Autodesk Fusion 360 part; units mm, degrees
sketch "Skizze1" plane through (0, 0, 0) normal (0, 0, 1) x (1, 0, 0)
  line L0 (-48.5045, 60.0252) -> (-48.5045, -50)
  line L1 (21.4307, 60.0126) -> (21.4307, -50)
  line L2 (-41.5077, 135.8568) -> (-13.5563, 144.0233)
  line L3 (-13.5563, 144.0233) -> (14.4793, 135.8568)
  line L4 (-41.4821, -125.8001) -> (-13.5254, -133.9377)
  line L5 (-13.5254, -133.9377) -> (14.4312, -125.8001)
  line L6 (14.4312, -125.8001) -> (14.4312, -57)
  line L7 (-41.4821, -125.8001) -> (-41.4821, -57)
  line L8 (-41.5077, 135.8568) -> (-41.5077, 66.6867)
  line L9 (14.4793, 135.8568) -> (14.4793, 66.6867)
  circle A0 centre (3.4202, 136.0177) radius 1.7651
  circle A1 centre (-30.4724, 136.0177) radius 1.7717
  circle A2 centre (-30.5621, -125.8912) radius 1.7405
  circle A3 centre (3.437, -125.8912) radius 1.7197
  circle A4 centre (-43.5796, -44.9629) radius 1.7343
  circle A5 centre (16.4191, -44.9629) radius 1.761
  circle A6 centre (-43.5796, 55.0289) radius 1.7075
  circle A7 centre (16.4191, 55.0289) radius 1.7507
  line L10 (21.4307, 60.0126) -> (21.4793, 60.0126)
  line L11 (14.4793, 67.0126) -> (14.4793, 66.6867)
  line L12 (-41.5077, 66.6867) -> (-41.5077, 67.0252)
  line L13 (-48.5077, 60.0252) -> (-48.5045, 60.0252)
  line L14 (-48.5045, -50) -> (-48.4821, -50)
  line L15 (21.4312, -50) -> (21.4307, -50)
  arc A8 (21.4312, -50) -> (14.4312, -57) centre (21.4312, -57) ccw
  arc A9 (-41.4821, -57) -> (-48.4821, -50) centre (-48.4821, -57) ccw
  arc A10 (-48.5077, 60.0252) -> (-41.5077, 67.0252) centre (-48.5077, 67.0252) ccw
  arc A11 (14.4793, 67.0126) -> (21.4793, 60.0126) centre (21.4793, 67.0126) ccw
  dimension "d1" = 7
  dimension "d2" = 7
  dimension "d3" = 7
  dimension "d4" = 7
extrude "Extrusion1" add sketch "Skizze1" along normal blind 3
sketch "Skizze2" plane through (0, 0, 0) normal (0, 0, 1) x (1, 0, 0)
  circle A0 centre (-13.6498, 118.1825) radius 1.7726
  circle A1 centre (-13.6498, 79.1243) radius 1.75
  circle A2 centre (-13.4454, 24.6727) radius 1.7602
  circle A3 centre (-13.5095, -14.2747) radius 1.7594
  circle A4 centre (-38.3105, 21.3875) radius 1.7537
  circle A5 centre (-38.3105, -36.6009) radius 1.7548
  circle A6 centre (11.0959, -36.6009) radius 1.7639
  circle A7 centre (11.0959, 21.3357) radius 1.7296
  circle A8 centre (-13.5725, -68.7537) radius 1.7556
  circle A9 centre (-13.5725, -107.7909) radius 1.7814
  dimension "d7" = 3.5
extrude "Extrusion2" cut sketch "Skizze2" along normal blind 10
sketch "Skizze3" plane through (0, 0, 3) normal (0, 0, 1) x (-1, 0, 0)
  circle A0 centre (13.6498, -118.1825) radius 1.7726
  circle A1 centre (38.3105, -21.3875) radius 1.7537
  circle A2 centre (38.3105, 36.6009) radius 1.7548
  circle A3 centre (13.4454, -24.6727) radius 1.7602
  circle A4 centre (13.5725, 107.7909) radius 1.7814
  circle A5 centre (13.6498, -79.1243) radius 1.75
  circle A6 centre (13.5095, 14.2747) radius 1.7594
  circle A7 centre (-11.0959, 36.6009) radius 1.7639
  circle A8 centre (-11.0959, -21.3357) radius 1.7296
  circle A9 centre (13.5725, 68.7537) radius 1.7556
  circle A10 centre (43.5796, 44.9629) radius 1.7343
  circle A11 centre (30.5621, 125.8912) radius 1.7405
  circle A12 centre (-16.4191, -55.0289) radius 1.7507
  circle A13 centre (-16.4191, 44.9629) radius 1.761
  circle A14 centre (30.4724, -136.0177) radius 1.7717
  circle A15 centre (-3.437, 125.8912) radius 1.7197
  circle A16 centre (-3.4202, -136.0177) radius 1.7651
  circle A17 centre (43.5796, -55.0289) radius 1.7075
  line L0 (41.5077, -135.8568) -> (41.5077, -67.0252)
  arc A18 (48.5045, -60.0252) -> (41.5077, -67.0252) centre (48.5077, -67.0252) ccw
  line L1 (48.5045, -60.0252) -> (48.5045, 50)
  line L2 (48.5045, 50) -> (48.4821, 50)
  arc A19 (41.4821, 57) -> (48.4821, 50) centre (48.4821, 57) ccw
  line L3 (41.4821, 57) -> (41.4821, 125.8001)
  line L4 (41.4821, 125.8001) -> (13.5254, 133.9377)
  line L5 (13.5254, 133.9377) -> (-14.4312, 125.8001)
  line L6 (-14.4312, 125.8001) -> (-14.4312, 57)
  arc A20 (-21.4307, 50) -> (-14.4312, 57) centre (-21.4312, 57) ccw
  line L7 (-21.4307, 50) -> (-21.4307, -60.0126)
  line L8 (-21.4307, -60.0126) -> (-21.4793, -60.0126)
  arc A21 (-14.4793, -67.0126) -> (-21.4793, -60.0126) centre (-21.4793, -67.0126) ccw
  line L9 (-14.4793, -67.0126) -> (-14.4793, -135.8568)
  line L10 (-14.4793, -135.8568) -> (13.5563, -144.0233)
  line L11 (13.5563, -144.0233) -> (41.5077, -135.8568)
  line L12 (48.4821, 50) -> (-21.4307, 50)
  line L13 (48.5045, -60.0252) -> (-21.4793, -60.0126)
  line L14 (-21.4793, -60.0126) -> (13.5127, -60.0126)
  line L15 (-21.4307, 50) -> (13.5257, 50)
  line L16 (-21.4307, 50) -> (13.5613, 50)
  line L17 (13.5127, -60.0126) -> (28.5127, -60.0153)
  line L18 (28.5127, -60.0153) -> (-1.4873, -60.0153)
  line L19 (13.5613, 50) -> (13.5613, 45)
  line L20 (13.5613, 45) -> (28.5613, 45)
  line L21 (28.5613, 45) -> (-1.4387, 45)
  line L22 (-1.4387, 45) -> (-1.4387, 55)
  line L23 (-1.4387, 55) -> (28.5613, 55)
  line L24 (28.5613, 55) -> (28.5613, 45)
  line L25 (-1.4873, -60.0153) -> (28.5127, -60.0153)
  line L26 (28.5127, -60.0153) -> (28.5127, -50.0153)
  line L27 (28.5127, -50.0153) -> (-1.4873, -50.0153)
  line L28 (-1.4873, -50.0153) -> (-1.4873, -60.0153)
  line L29 (-1.4387, 45) -> (28.5613, 45)
  line L30 (28.5613, 45) -> (28.5613, 40)
  line L31 (28.5613, 40) -> (-1.4387, 40)
  line L32 (-1.4387, 40) -> (-1.4387, 45)
  line L33 (-1.4873, -50.0153) -> (28.5127, -50.0153)
  line L34 (28.5127, -50.0153) -> (28.5127, -45.0153)
  line L35 (28.5127, -45.0153) -> (-1.4873, -45.0153)
  line L36 (-1.4873, -45.0153) -> (-1.4873, -50.0153)
  dimension "d10" = 34.992
  dimension "d11" = 34.992
  dimension "d12" = 15
  dimension "d13" = 30
  dimension "d15" = 5
  dimension "d16" = 15
  dimension "d17" = 30
  dimension "d18" = 10
  dimension "d19" = 30
  dimension "d20" = 10
  dimension "d21" = 30
  dimension "d22" = 5
  dimension "d23" = 30
  dimension "d24" = 5
extrude "Extrusion3" cut sketch "Skizze3" against normal blind 10 contours L14 L17 L26 L27 L28 L33 | L27 L33 L34 L35 L36 | L12 L19 L20 L21 L24 L29 | L12 L15 L16 L22 L23 L24 | L12 L15 L16 L19 L21 L22 L29 | L20 L21 L29 L30 L31 L32
Build history of the part. All positions in model axes, mm. Round coordinates to 2 decimals unless told otherwise and drop trailing zeros. Write each loop counter-clockwise with the first axis right and the second up, starting at its lowest first coordinate (ties: lowest second). Pieces come first, ordered by that corner, then holes. Notation, with made-up numbers: (57.5, -6) - (116.5, -6) arc R22 ccw to (116.5, 11) - close; hole circle Ø10 at (-19.5, 33.25). An arc over 180 degrees is marked (long way). One line per question, with ' | ' between items.
1. Band-saw the part on B-B, the plane y = 127. Write the cut outline in (x, z).
Results are:
outline: (-41.51, 0) - (14.48, 0) - (14.48, 3) - (-41.51, 3) - close
2. Band-saw the part on C-C, the plane z = 0.6. Give the number of separate pieces and of enclosed holes in the cut face, and give its area (3 significant figures).
Results are:
separate pieces: 1 | enclosed holes: 20 | area: 15,600 mm^2
3. Band-saw the part on A-A, the plane y = 48.5. Write the cut outline in (x, z), and give its area (3 significant figures).
Results are:
outline: (-48.5, 0) - (-28.51, 0) - (-28.51, 3) - (-48.5, 3) - close; (1.49, 0) - (21.43, 0) - (21.43, 3) - (1.49, 3) - close | area: 120 mm^2
4. Drill centre lines: line 1 along Y through (x, z) = (-16, 2.25); line 2 along Y through (x, z) = (-6, 0.9); line 3 along X through (y, z) = (-14.5, 1.1). Where is each one in solid material? Low to high. Write a range as from..to.
Results are:
line 1: -133.22..-55, -40..45.02, 60.01..143.31 | line 2: -131.75..-55, -40..45.02, 60.01..141.82 | line 3: -48.5..-15.25, -11.76..21.43
5. Drop flat-ended pins along their axis: pin 1 Ø3 at (x, y) = (11.1, -36.6) entering from +Z (3 decimals); pin 2 Ø1.5 at (x, z) = (-8, 1.5) entering from -Y; pin 3 Ø1.5 at (y, z) = (102.5, 2) entering from +X; pin 4 Ø1.5 at (y, z) = (-79.5, 1) entering from -X. Give the stop position or say it passes through.
Results are:
pin 1: through | pin 2: y = -132.55 | pin 3: x = 14.48 | pin 4: x = -41.48
